For this review, take the finished solid that the model builds, in its own axes (mm). A direction names the side the tool comes from. Give positions to 0.01 mm unless a question says otherwise; leave off trailing zeros. Loops run counter-clockwise (first coordinate to the right, second up) from the corner with the lowest first, then second, coordinate; pieces in that order, holes last.
```python
from build123d import *

# Parameters (mm, degrees)
SKETCH1_W           = 10
SKETCH1_H           = 10
BOSS_EXTRUDE1_DEPTH = 56.642
SKETCH3_R           = 1.35
CUT_EXTRUDE1_DEPTH  = 10
SKETCH4_R           = 1.35
CUT_EXTRUDE2_DEPTH  = 7
SKETCH8_R           = 1.48
CUT_EXTRUDE3_DEPTH  = 6


with BuildPart() as part:
    # Sketch1 → Boss-Extrude1 (new body)
    with BuildSketch(Plane(origin=(0, 0, 0), x_dir=(1, 0, 0), z_dir=(0, 1, 0))):
        with Locations((1.057692308, -0.576923077)):
            Rectangle(SKETCH1_W, SKETCH1_H)
    extrude(amount=BOSS_EXTRUDE1_DEPTH)

    # Sketch3 → Cut-Extrude1 (cut)
    with BuildSketch(Plane.XY.offset(5.576923077)):
        with Locations((1.137692308, 19.05)):
            Circle(SKETCH3_R)
        with Locations((1.137692308, 52.832)):
            Circle(SKETCH3_R)
    extrude(amount=-CUT_EXTRUDE1_DEPTH, mode=Mode.SUBTRACT)

    # Sketch4 → Cut-Extrude2 (cut)
    with BuildSketch(Plane.ZY.offset(3.942307692)):
        with Locations((0.576923077, 12.690710938)):
            Circle(SKETCH4_R)
        with Locations((0.576923077, 46.642)):
            Circle(SKETCH4_R)
    extrude(amount=-CUT_EXTRUDE2_DEPTH, mode=Mode.SUBTRACT)

    # Sketch8 → Cut-Extrude3 (cut)
    with BuildSketch(Plane(origin=(0, 0, 0), x_dir=(-1, 0, 0), z_dir=(0, -1, 0))):
        with Locations(Location((-0.977692308, -0.496923077, 0), (0, 0, 90))):
            Circle(SKETCH8_R)
    extrude(amount=-CUT_EXTRUDE3_DEPTH, mode=Mode.SUBTRACT)


solid = part.part
```
Q1. Mouldability with a two-part tool opening along X and no side actions: class faces 4 (the cylindrical face through (1.76, 17.85, 0.65)), 5 (the flat face through (1, 28, 5.577)), 6 (the flat face through (3.058, 47, 1)) as +X half, -X half, draft (parallel to the pull), parting line (faces both ways), or undercut.
Answers:
face 4: undercut
face 5: draft
face 6: -X half
Q2. Machinability: for faces 1 (the cylindrical face through (2.445, 2.958, 0.69)), 2 (the flat face through (1, 28, -4.423)), 3 (the cylindrical face through (-0.49, 47.98, 0.4)), which of the approach directions +Z, -Z, +X, -X, +Y, -Y give a long, thin tool a straight path to every point of the face, cutting with its end or side? Answer none if there is none.
Answers:
face 1: -Y
face 2: -Z, +X, -X, +Y, -Y
face 3: -X
Q3. For probe 1 along Y at (x, z) = (2, -0.5); probe 2 along Y at (x, z) = (-1, -0.25); probe 3 along Y at (x, z) = (1.75, -2), list the stretches that pass through material, from the lowest coordinate up.
Answers:
probe 1: y = 6 to 11.88, 13.5 to 18.01, 20.09 to 45.83, 47.46 to 51.79, 53.87 to 56.64
probe 2: y = 0 to 11.62, 13.76 to 45.57, 47.71 to 56.64
probe 3: y = 0 to 17.85, 20.25 to 51.63, 54.04 to 56.64
Q4. Consider section A-A on y = 19.05. Give the boundary of the cut face in (x, z), plus the area to 3 significant figures.
Answers:
outline: (-3.94, -4.42) - (-0.21, -4.42) - (-0.21, 5.58) - (-3.94, 5.58) - close; (2.49, -4.42) - (6.06, -4.42) - (6.06, 5.58) - (2.49, 5.58) - close
area: 73.0 mm2
Q5. For pin 1 Ø1.3 at (y, z) = (12.5, 1) entering from -X; pin 2 Ø3.5 at (x, y) = (1.14, 52.83) entering from +Z; pin 3 Ø2.5 at (x, y) = (1.14, 19.05) entering from +Z, all flat-tipped, find the tip position at first contact; note any pin that passes through.
Answers:
pin 1: stops at x = 3.06
pin 2: stops at z = 5.58
pin 3: passes through
Q6. Consider section B-B on z = 1. Give the boundary of the cut face in (x, y).
Answers:
outline: (-3.94, 0) - (-0.41, 0) - (-0.41, 6) - (2.37, 6) - (2.37, 0) - (6.06, 0) - (6.06, 56.64) - (-3.94, 56.64) - (-3.94, 47.92) - (3.06, 47.92) - (3.06, 45.36) - (-3.94, 45.36) - (-3.94, 13.97) - (3.06, 13.97) - (3.06, 11.41) - (-3.94, 11.41) - close; hole circle Ø2.7 at (1.14, 19.05); hole circle Ø2.7 at (1.14, 52.83)
Q7. Consider section D-D on z = 4.25. Give the boundary of the cut face in (x, y), plus the area to 3 significant figures.
Answers:
outline: (-3.94, 0) - (6.06, 0) - (6.06, 56.64) - (-3.94, 56.64) - close; hole circle Ø2.7 at (1.14, 19.05); hole circle Ø2.7 at (1.14, 52.83)
area: 555 mm2
Q8. Consider section C-C on x = -3. Give the boundary of the cut face in (y, z), plus the area to 3 significant figures.
Answers:
outline: (0, -4.42) - (56.64, -4.42) - (56.64, 5.58) - (0, 5.58) - close; hole circle Ø2.7 at (12.69, 0.58); hole circle Ø2.7 at (46.64, 0.58)
area: 555 mm2
